The listing builds one solid part. Answer for the finished solid, in the listing's coordinates (mm). Coordinates: 2 decimals unless noted, no trailing zeros. Order: outer loops, then holes, each group sorted by start corner. A loop starts at its lowest first (then second) coordinate and runs counter-clockwise, first axis right, second up. Notation, with made-up numbers: (-39.75, 41) -> (10.25, 41) arc R16 cw to (10.25, 56) -> close; hole circle Ø2 at (87, -6.75). An arc over 180 degrees is marked (long way). Write item = value, one per line.
from build123d import *

# Parameters (mm, degrees)
SKETCH_2_R        = 0.4
EXTRUDE_1_DEPTH   = 3
EXTRUDE_1_2_DEPTH = 3
EXTRUDE_1_3_DEPTH = 3
EXTRUDE_1_4_DEPTH = 3
EXTRUDE_1_5_DEPTH = 3
EXTRUDE_2_DEPTH   = 12.7
FILLET_1_R        = 1


with BuildPart() as part:
    # Sketch 2 → Extrude 1 (new body)
    with BuildSketch(Plane(origin=(0, 0, 0), x_dir=(1, 0, 0), z_dir=(0, 1, 0))):
        with Locations(Location((0, 0, 0), (0, 0, 270))):
            Circle(SKETCH_2_R)
    extrude(amount=-EXTRUDE_1_DEPTH)



with BuildPart() as body_2:
    # Sketch 2 → Extrude 1 2 (new body)
    with BuildSketch(Plane(origin=(0, 0, 0), x_dir=(1, 0, 0), z_dir=(0, 1, 0))):
        with Locations(Location((9.525, 0, 0), (0, 0, 270))):
            Circle(SKETCH_2_R)
    extrude(amount=-EXTRUDE_1_2_DEPTH)


with BuildPart() as body_3:
    # Sketch 2 → Extrude 1 3 (new body)
    with BuildSketch(Plane(origin=(0, 0, 0), x_dir=(1, 0, 0), z_dir=(0, 1, 0))):
        with Locations(Location((0, -19.05, 0), (0, 0, 270))):
            Circle(SKETCH_2_R)
    extrude(amount=-EXTRUDE_1_3_DEPTH)


with BuildPart() as body_4:
    # Sketch 2 → Extrude 1 4 (new body)
    with BuildSketch(Plane(origin=(0, 0, 0), x_dir=(1, 0, 0), z_dir=(0, 1, 0))):
        with Locations(Location((19.05, -19.05, 0), (0, 0, 270))):
            Circle(SKETCH_2_R)
    extrude(amount=-EXTRUDE_1_4_DEPTH)


with BuildPart() as body_5:
    # Sketch 2 → Extrude 1 5 (new body)
    with BuildSketch(Plane(origin=(0, 0, 0), x_dir=(1, 0, 0), z_dir=(0, 1, 0))):
        with Locations(Location((19.05, 0, 0), (0, 0, 270))):
            Circle(SKETCH_2_R)
    extrude(amount=-EXTRUDE_1_5_DEPTH)


with BuildPart() as part_1:
    add(part.part)

    add(body_2.part)  # Extrude 2 merges body 2

    add(body_3.part)  # Extrude 2 merges body 3

    add(body_4.part)  # Extrude 2 merges body 4

    add(body_5.part)  # Extrude 2 merges body 5
    # Sketch 3 → Extrude 2 (add)
    with BuildSketch(Plane(origin=(0, 0, 0), x_dir=(1, 0, 0), z_dir=(0, 1, 0))):
        with BuildLine():
            Line((-2.175, 3.175), (21.225, 3.175))
            ThreePointArc((21.225, 3.175), (21.932106781, 2.882106781), (22.225, 2.175))
            Line((22.225, 2.175), (22.225, -21.225))
            ThreePointArc((22.225, -21.225), (21.932106781, -21.932106781), (21.225, -22.225))
            Line((21.225, -22.225), (-2.175, -22.225))
            ThreePointArc((-2.175, -22.225), (-2.882106781, -21.932106781), (-3.175, -21.225))
            Line((-3.175, -21.225), (-3.175, 2.175))
            ThreePointArc((-3.175, 2.175), (-2.882106781, 2.882106781), (-2.175, 3.175))
        make_face()
    extrude(amount=EXTRUDE_2_DEPTH)

    # Fillet 1
    fillet_1_edges = [part_1.edges().sort_by_distance(p)[0] for p in [
        (22.225, 12.7, 9.525),
        (21.932106781, 12.7, -2.882106781),
        (9.525, 12.7, -3.175),
        (-2.882106781, 12.7, -2.882106781),
        (-3.175, 12.7, 9.525),
        (-2.882106781, 12.7, 21.932106781),
        (9.525, 12.7, 22.225),
        (21.932106781, 12.7, 21.932106781),
    ]]
    fillet(fillet_1_edges, radius=FILLET_1_R)


solid = part_1.part
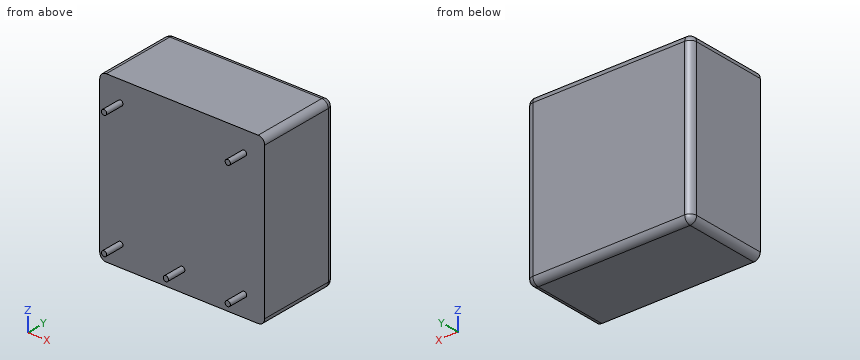
Q1. This flat-tipped pin is pushed along its axis until it touches: pin 1 Ø7.5 at (x, z) = (11.5, 6) entering from -Y. Where does it stop, or does it pass through?
The answers:
pin_1 = 0
Q2. Find the intervals of material crossed by line 1 along Y through (x, z) = (18, 20.5); line 2 along Z through (x, y) = (18.75, -1.75); line 3 along X through (y, z) = (12.25, 18.5), in increasing order.
The answers:
line_1 = 0 to 12.7
line_2 = -0.26 to 0.26, 18.79 to 19.31
line_3 = -3.01 to 22.06
Q3. Section C-C, the plane y = -1.25 is taken. Give the vertices of the cut face in (x, z) (3 decimals), plus the area to 3 significant figures.
The answers:
outline = circle Ø0.8 at (0, 0); circle Ø0.8 at (0, 19.05); circle Ø0.8 at (9.525, 0); circle Ø0.8 at (19.05, 0); circle Ø0.8 at (19.05, 19.05)
area = 2.51 mm2
Q4. Section A-A, the plane x = 0 is taken. Give the vertices of the cut face in (y, z) (3 decimals), plus the area to 3 significant figures.
The answers:
outline = (-3, -0.4) -> (0, -0.4) -> (0, -3.175) -> (11.7, -3.175) arc R1 ccw to (12.7, -2.175) -> (12.7, 21.225) arc R1 ccw to (11.7, 22.225) -> (0, 22.225) -> (0, 19.45) -> (-3, 19.45) -> (-3, 18.65) -> (0, 18.65) -> (0, 0.4) -> (-3, 0.4) -> close
area = 327 mm2
Q5. Section D-D, the plane z = 19.05 is taken. Give the vertices of the cut face in (x, y) (3 decimals).
The answers:
outline = (-3.175, 0) -> (-0.4, 0) -> (-0.4, -3) -> (0.4, -3) -> (0.4, 0) -> (18.65, 0) -> (18.65, -3) -> (19.45, -3) -> (19.45, 0) -> (22.225, 0) -> (22.225, 11.7) arc R1 ccw to (21.225, 12.7) -> (-2.175, 12.7) arc R1 ccw to (-3.175, 11.7) -> close
Q6. Section B-B, the plane z = 3.75 is taken. Give the vertices of the cut face in (x, y) (3 decimals).
The answers:
outline = (-3.175, 0) -> (22.225, 0) -> (22.225, 11.7) arc R1 ccw to (21.225, 12.7) -> (-2.175, 12.7) arc R1 ccw to (-3.175, 11.7) -> close
